Can you work these out from the model? Positions are in its coordinate system, mm. Face numbers are marked on the shaded views. Round coordinates to 2 decimals unless told otherwise and drop trailing zeros. Loops run counter-clockwise (first coordinate to the right, second up) from the corner with the lowest first, then second, coordinate; pieces in that order, holes last.
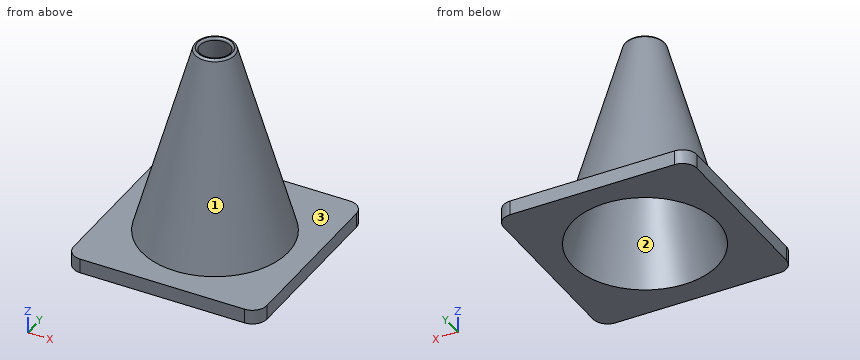
from build123d import *

# Parameters (mm, degrees)
FILLET001_R = 0.4
FILLET002_R = 0.5
BOX_W       = 40
BOX_H       = 40
BOX_DEPTH   = 3
FILLET_R    = 3


with BuildPart() as cono_interior:
    # Cone001 → Cone001 (revolve)
    with BuildSketch(Plane(origin=(20, 20, 0), x_dir=(1, 0, 0), z_dir=(0, -1, 0))):
        Polygon((0, 0), (15, 0), (3, 43), (0, 43), align=None)
    revolve(axis=Axis((20, 20, 0), (0, 0, 1)))


with BuildPart() as obj1:
    # Cone → Cone (revolve)
    with BuildSketch(Plane(origin=(20, 20, 0), x_dir=(1, 0, 0), z_dir=(0, -1, 0))):
        Polygon((0, 0), (16, 0), (4, 43), (0, 43), align=None)
    revolve(axis=Axis((20, 20, 0), (0, 0, 1)))

    # Cut: cut cono_interior
    add(cono_interior.part, mode=Mode.SUBTRACT)

    # Fillet001
    fillet001_edges = [obj1.edges().sort_by_distance(p)[0] for p in [
        (17, 20, 43),
    ]]
    fillet(fillet001_edges, radius=FILLET001_R)

    # Fillet002
    fillet002_edges = [obj1.edges().sort_by_distance(p)[0] for p in [
        (16, 20, 43),
    ]]
    fillet(fillet002_edges, radius=FILLET002_R)


with BuildPart() as cono_final:
    # Box → Box (new body)
    with BuildSketch(Plane.XY):
        with Locations((20, 20)):
            Rectangle(BOX_W, BOX_H)
    extrude(amount=BOX_DEPTH)

    # Fillet
    fillet_edges = [cono_final.edges().sort_by_distance(p)[0] for p in [
        (0, 0, 1.5),
        (0, 40, 1.5),
        (40, 0, 1.5),
        (40, 40, 1.5),
    ]]
    fillet(fillet_edges, radius=FILLET_R)

    # Cut001: cut cono_interior
    add(cono_interior.part, mode=Mode.SUBTRACT)

    # Fusion: union obj1
    add(obj1.part)


solid = cono_final.part
(1) If I drill on line 1 (Z direction, x = 5.5, y = 38); line 2 (X direction, y = 23, z = 27.5); line 3 (Y direction, x = 26.5, z = 17), over which ranges is the centre line in solid material (lowest first)?
Worked answers:
line 1: z = 0 to 3
line 2: x = 12.23 to 13.32, 26.68 to 27.77
line 3: y = 10.81 to 12.07, 27.93 to 29.19
(2) If we mould it in two halves opening along X, with no side actions, what happens to the marked faces 1, 2 and 3? For each: released by +X, released by -X, zero draft, split by the parting line, or undercut.
Worked answers:
face 1: split by the parting line
face 2: undercut
face 3: zero draft
(3) If we section it at C-C, the plane z = 4.5: List the corners of the cut face in (x, y) for me.
Worked answers:
outline: circle Ø29.49 at (20, 20); hole circle Ø27.49 at (20, 20)
(4) Will these pins go through, and if not, where does the flat tip stop? P1, Ø5, axis at y = 10, z = 27.5, coming from the -X side; P2, Ø2, axis at y = 20, z = 20, coming from the -X side; P3, Ø2, axis at x = 16.5, z = 35.5, coming from the -Y side.
Worked answers:
P1: stops at x = 16.15
P2: stops at x = 9.3
P3: stops at y = 14.35
(5) If we section it at D-D, the plane z = 20: List the corners of the cut face in (x, y) for me, then the cut area to 3 significant figures.
Worked answers:
outline: circle Ø20.84 at (20, 20); hole circle Ø18.84 at (20, 20)
area: 62.3 mm2
(6) If we section it at A-A, the plane y = 20: List the corners of the cut face in (x, z) for me, then the cut area to 3 significant figures.
Worked answers:
outline: (0, 0) - (5, 0) - (16.86, 42.49) arc R0.4 ccw to (16.47, 43) - (16.38, 43) arc R0.5 ccw to (15.9, 42.63) - (4.84, 3) - (0, 3) - close; (23.14, 42.49) - (35, 0) - (40, 0) - (40, 3) - (35.16, 3) - (24.1, 42.63) arc R0.5 ccw to (23.62, 43) - (23.53, 43) arc R0.4 ccw to start
area: 112 mm2
